Input: dimensioned drawing with shaded views. Units: mm. Origin: part minimum x, y, z. Round coordinates to 2 decimals unless told otherwise and drop trailing zeros. Loops run counter-clockwise (first coordinate to the right, second up) from the corner with the lowest first, then second, coordinate; pieces in that order, holes last. Notation, with made-up numbers: M -3,23 L 47,23 A7 cw 47,31 Z; hole C -8.5,69 d7. An arc over 180 degrees is marked long. Answer as a JSON object with one key per item and string values.
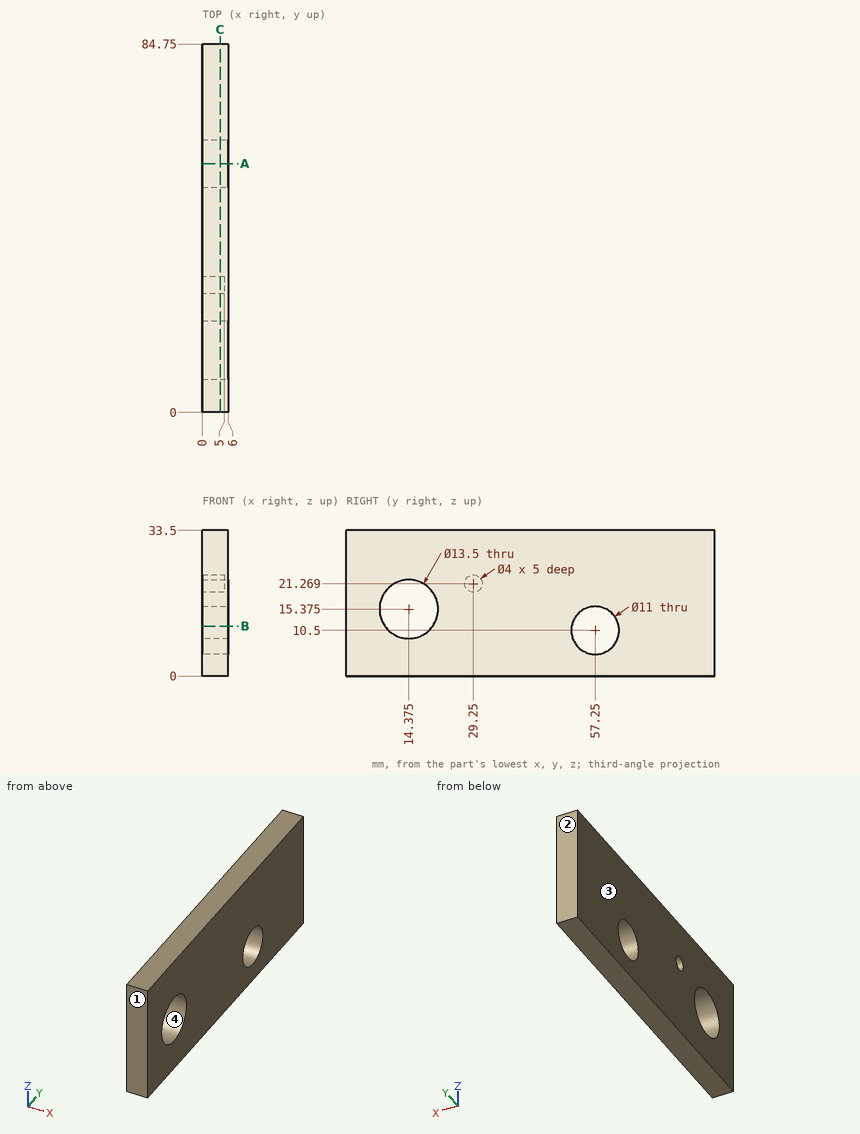
Item 1: Section C-C on x = 4.1. Give the number of separate pieces and of enclosed holes in the cut face, then the cut area to 3 significant figures.
Answer sheet:
{"separate pieces": "1", "enclosed holes": "3", "area": "2,590 mm²"}
Item 2: Contact query for a flat-ended pin moving along its axis: pin 1 Ø9 at (y, z) = (57.25, 10.5) entering from -X. Output: stop coordinate, or through.
Answer sheet:
{"pin 1": "passes through"}
Item 3: Section B-B on z = 11.5. Return the cut outline in (x, y), then the cut area to 3 significant figures.
Answer sheet:
{"outline": "M 0,0 L 6,0 L 6,8.85 L 0,8.85 Z; M 0,19.9 L 6,19.9 L 6,51.84 L 0,51.84 Z; M 0,62.66 L 6,62.66 L 6,84.75 L 0,84.75 Z", "area": "377 mm²"}
Item 4: Pull-direction query (Y, two-part tool) for the marked faces 1, 2, 3 and 4; classes: pulls with the +Y half, pulls with the -Y half, needs draft (parallel to the pull), parting line crosses it, or undercut.
Answer sheet:
{"face 1": "pulls with the -Y half", "face 2": "pulls with the +Y half", "face 3": "needs draft", "face 4": "undercut"}
Item 5: Line query: probe 1 along Z at (x, y) = (1.9, 14.5); probe 2 along Y at (x, z) = (4.7, 12); probe 3 along Z at (x, y) = (2.8, 61.5). Output: solid intervals per line, ascending. Write a range as from..to.
Answer sheet:
{"probe 1": "z = 0..8.63, 22.12..33.5", "probe 2": "y = 0..8.53, 20.22..51.96, 62.54..84.75", "probe 3": "z = 0..7.01, 13.99..33.5"}
Item 6: Section A-A on y = 57.25. Return the cut outline in (x, z), then the cut area to 3 significant figures.
Answer sheet:
{"outline": "M 0,0 L 6,0 L 6,5 L 0,5 Z; M 0,16 L 6,16 L 6,33.5 L 0,33.5 Z", "area": "135 mm²"}
